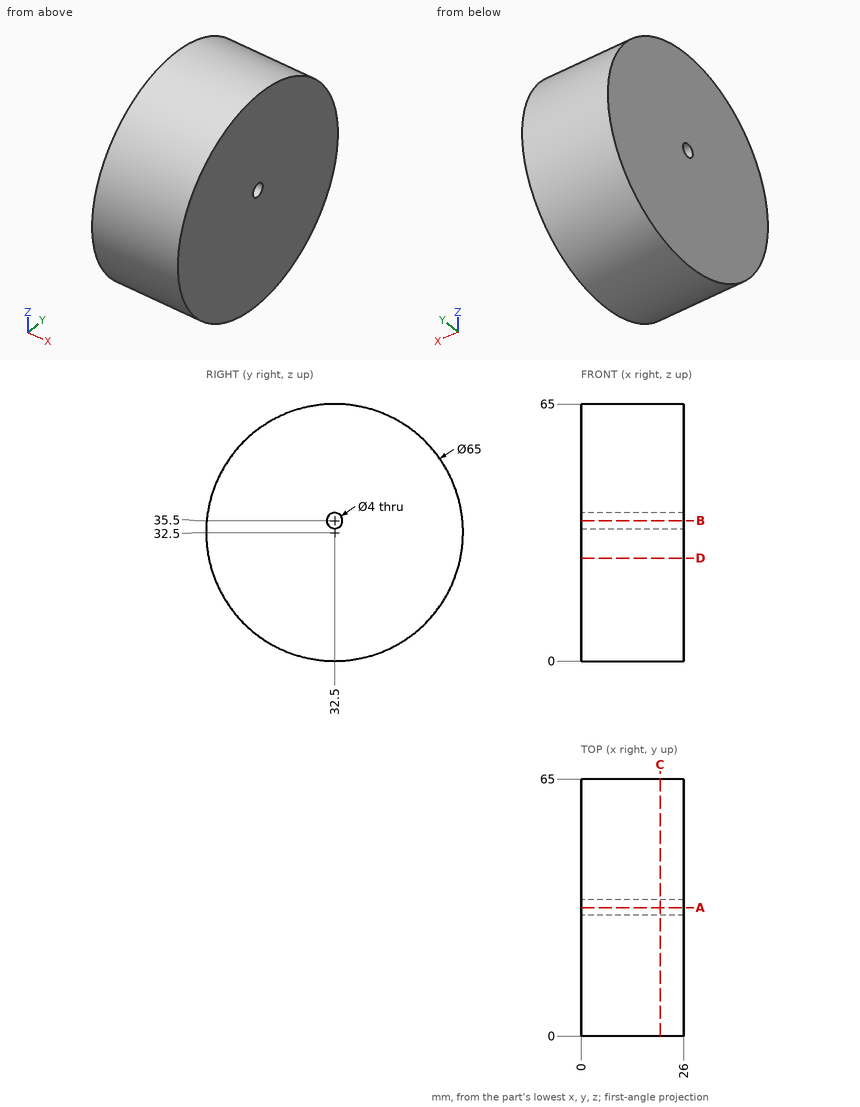
The drawing under review shows one solid part. Ordinate dimensions are in mm from its lowest x, y, z. Coordinates: 2 decimals unless noted, no trailing zeros. Loops run counter-clockwise (first coordinate to the right, second up) from the corner with the lowest first, then second, coordinate; pieces in that order, holes last. Notation, with made-up numbers: (-34, -23) - (21, -23) arc R28 cw to (21, 5) - close; hole circle Ø2 at (24.5, 86). An arc over 180 degrees is marked (long way). Use CSV: the item, a comma, the result in double quotes. Start each with the question number.
1. Add section D-D on z = 26. Give the boundary of the cut face in (x, y).
2. To check wall thickness, follow probe 1 along Y at (x, z) = (14.25, 35.5); probe 2 along Z at (x, y) = (2.75, 51.5); probe 3 along Y at (x, z) = (17, 58). State the ranges of each line that lie inside material, in increasing order.
3. Add section A-A on y = 32.5. Give the boundary of the cut face in (x, z), plus the area to 3 significant figures.
4. Add section C-C on x = 20. Give the boundary of the cut face in (y, z), plus the area to 3 significant figures.
5. Add section B-B on z = 35.5. Give the boundary of the cut face in (x, y).
6. Clearance check with flat-ended pins moving along their axes: pin 1 (8 mm diameter, centred on x = 16, y = 26, fed in from -Z); pin 2 (12 mm diameter, centred on x = 21.5, z = 25, fed in from +Y); pin 3 (3 mm diameter, centred on x = 10.5, y = 30, fed in from +Z). State where each tip first meets the part, or that it passes through.
Resolved:
1,outline,"(0, 0.66) - (26, 0.66) - (26, 64.34) - (0, 64.34) - close"
2,probe 1,"0.14 to 30.5, 34.5 to 64.86"
2,probe 2,"6.13 to 58.87"
2,probe 3,"12.35 to 52.65"
3,outline,"(0, 0) - (26, 0) - (26, 33.5) - (0, 33.5) - close; (0, 37.5) - (26, 37.5) - (26, 65) - (0, 65) - close"
3,area,"1,590 mm2"
4,outline,"circle Ø65 at (32.5, 32.5); hole circle Ø4 at (32.5, 35.5)"
4,area,"3,310 mm2"
5,outline,"(0, 0.14) - (26, 0.14) - (26, 30.5) - (0, 30.5) - close; (0, 34.5) - (26, 34.5) - (26, 64.86) - (0, 64.86) - close"
6,pin 1,"z = 0.1"
6,pin 2,"y = 64.97"
6,pin 3,"z = 64.98"
